from build123d import *

# Parameters (mm, degrees)
SKETCH1_W           = 90
SKETCH1_H           = 30
BOSS_EXTRUDE1_DEPTH = 5.9
SKETCH2_R           = 2.75
CUT_EXTRUDE1_DEPTH  = 10
SKETCH3_W           = 5.9
SKETCH3_H           = 10
CUT_EXTRUDE2_DEPTH  = 10
CUT_EXTRUDE5_REACH  = 7.9
SKETCH6_R           = 2.05
FILLET1_R           = 12
FILLET1_2_R         = 6


with BuildPart() as part:
    # Sketch1 → Boss-Extrude1 (new body)
    with BuildSketch(Plane(origin=(0, 0, 0), x_dir=(1, 0, 0), z_dir=(0, 1, 0))):
        Rectangle(SKETCH1_W, SKETCH1_H)
    extrude(amount=BOSS_EXTRUDE1_DEPTH)

    # Sketch2 → Cut-Extrude1 (cut)
    with BuildSketch(Plane(origin=(0, 5.9, 0), x_dir=(1, 0, 0), z_dir=(0, 1, 0))):
        with Locations((25, 0)):
            Circle(SKETCH2_R)
        with Locations((-38, 0)):
            Circle(SKETCH2_R)
    extrude(amount=-CUT_EXTRUDE1_DEPTH, mode=Mode.SUBTRACT)

    # Sketch3 → Cut-Extrude2 (cut)
    with BuildSketch(Plane(origin=(0, 5.9, 0), x_dir=(1, 0, 0), z_dir=(0, 1, 0))):
        with Locations((-2.95, 0)):
            Rectangle(SKETCH3_W, SKETCH3_H)
    extrude(amount=-CUT_EXTRUDE2_DEPTH, mode=Mode.SUBTRACT)

    # Sketch6 → Cut-Extrude5 (cut, up to next)
    with BuildSketch(Plane(origin=(0, 5.9, 0), x_dir=(1, 0, 0), z_dir=(0, 1, 0)), mode=Mode.PRIVATE) as cut_extrude5_sk1:
        with Locations((0, 5)):
            Circle(SKETCH6_R)
    cut_extrude5_tool1 = extrude(cut_extrude5_sk1.sketch, amount=-CUT_EXTRUDE5_REACH, mode=Mode.PRIVATE) & part.part
    add(cut_extrude5_tool1.solids().sort_by_distance((0, 5.9, -5))[0], mode=Mode.SUBTRACT)
    # Sketch6 → Cut-Extrude5 (cut, up to next)
    with BuildSketch(Plane(origin=(0, 5.9, 0), x_dir=(1, 0, 0), z_dir=(0, 1, 0)), mode=Mode.PRIVATE) as cut_extrude5_sk2:
        with Locations((-5.9, 5)):
            Circle(SKETCH6_R)
    cut_extrude5_tool2 = extrude(cut_extrude5_sk2.sketch, amount=-CUT_EXTRUDE5_REACH, mode=Mode.PRIVATE) & part.part
    add(cut_extrude5_tool2.solids().sort_by_distance((-5.9, 5.9, -5))[0], mode=Mode.SUBTRACT)
    # Sketch6 → Cut-Extrude5 (cut, up to next)
    with BuildSketch(Plane(origin=(0, 5.9, 0), x_dir=(1, 0, 0), z_dir=(0, 1, 0)), mode=Mode.PRIVATE) as cut_extrude5_sk3:
        with Locations((0, -5)):
            Circle(SKETCH6_R)
    cut_extrude5_tool3 = extrude(cut_extrude5_sk3.sketch, amount=-CUT_EXTRUDE5_REACH, mode=Mode.PRIVATE) & part.part
    add(cut_extrude5_tool3.solids().sort_by_distance((0, 5.9, 5))[0], mode=Mode.SUBTRACT)
    # Sketch6 → Cut-Extrude5 (cut, up to next)
    with BuildSketch(Plane(origin=(0, 5.9, 0), x_dir=(1, 0, 0), z_dir=(0, 1, 0)), mode=Mode.PRIVATE) as cut_extrude5_sk4:
        with Locations((-5.9, -5)):
            Circle(SKETCH6_R)
    cut_extrude5_tool4 = extrude(cut_extrude5_sk4.sketch, amount=-CUT_EXTRUDE5_REACH, mode=Mode.PRIVATE) & part.part
    add(cut_extrude5_tool4.solids().sort_by_distance((-5.9, 5.9, 5))[0], mode=Mode.SUBTRACT)

    # Fillet1
    fillet1_edges = [part.edges().sort_by_distance(p)[0] for p in [
        (-45, 2.95, -15),
        (-45, 2.95, 15),
    ]]
    fillet(fillet1_edges, radius=FILLET1_R)

    # Fillet1 2
    fillet1_2_edges = [part.edges().sort_by_distance(p)[0] for p in [
        (45, 2.95, 15),
        (45, 2.95, -15),
    ]]
    fillet(fillet1_2_edges, radius=FILLET1_2_R)


solid = part.part
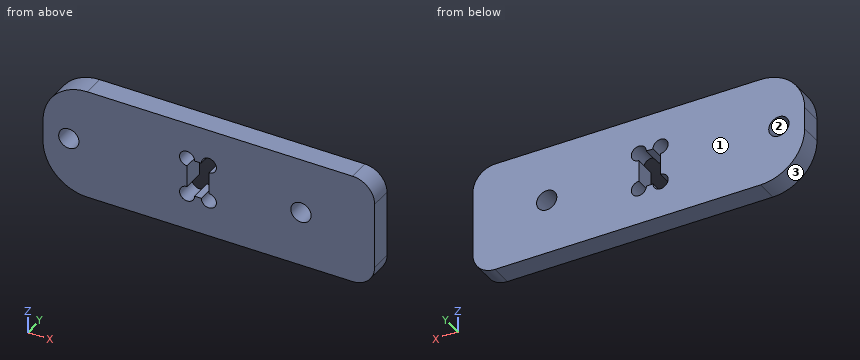
The listing builds one solid part. Answer for the finished solid, in the listing's coordinates (mm). Face numbers are marked on the shaded views. Coordinates: 2 decimals unless noted, no trailing zeros. Write each loop counter-clockwise with the first axis right and the second up, starting at its lowest first coordinate (ties: lowest second). Pieces come first, ordered by that corner, then holes. Notation, with made-up numbers: (-16, 66.5) -> (15, 66.5) arc R17 ccw to (15, 87.5) -> close; hole circle Ø2 at (27.25, -29). An arc over 180 degrees is marked (long way). One line per question, with ' | ' between items.
1. Section B-B (z = 1.5) is taken. Determine the outline of the cut face in (x, y).
Verdict:
outline: (-45, 0) -> (-40.3, 0) -> (-40.3, 5.9) -> (-45, 5.9) -> close; (-35.7, 0) -> (-5.9, 0) -> (-5.9, 5.9) -> (-35.7, 5.9) -> close; (0, 0) -> (22.7, 0) -> (22.7, 5.9) -> (0, 5.9) -> close; (27.3, 0) -> (45, 0) -> (45, 5.9) -> (27.3, 5.9) -> close
2. Section A-A (y = 1.8) is taken. Determine the outline of the cut face in (x, z).
Verdict:
outline: (-45, -3) arc R12 ccw to (-33, -15) -> (39, -15) arc R6 ccw to (45, -9) -> (45, 9) arc R6 ccw to (39, 15) -> (-33, 15) arc R12 ccw to (-45, 3) -> close; hole circle Ø5.5 at (-38, 0); hole (-5.9, -2.95) arc R2.05 ccw (long way) to (-3.85, -5) -> (-2.05, -5) arc R2.05 ccw (long way) to (0, -2.95) -> (0, 2.95) arc R2.05 ccw (long way) to (-2.05, 5) -> (-3.85, 5) arc R2.05 ccw (long way) to (-5.9, 2.95) -> close; hole circle Ø5.5 at (25, 0)
3. Section C-C (x = -38) is taken. Determine the outline of the cut face in (y, z).
Verdict:
outline: (0, -13.91) -> (5.9, -13.91) -> (5.9, -2.75) -> (0, -2.75) -> close; (0, 2.75) -> (5.9, 2.75) -> (5.9, 13.91) -> (0, 13.91) -> close
4. For a pull along Z with two mould halves and no side action, classify the marked faces 1, 2 and 3 as released by +Z, released by -Z, zero draft, split by the parting line, or undercut.
Verdict:
face 1: zero draft | face 2: undercut | face 3: released by -Z
5. Section D-D (z = 6) is taken. Determine the outline of the cut face in (x, y).
Verdict:
outline: (-44.62, 0) -> (-7.69, 0) -> (-7.69, 5.9) -> (-44.62, 5.9) -> close; (-4.11, 0) -> (-1.79, 0) -> (-1.79, 5.9) -> (-4.11, 5.9) -> close; (1.79, 0) -> (45, 0) -> (45, 5.9) -> (1.79, 5.9) -> close
6. Straight lines are drawn through the part: line 1 (X direction, y = 2.85, z = 0); line 2 (X direction, y = 1.95, z = -6.5); line 3 (X direction, y = 3.9, z = -4.5). For each, find the intervals that lie inside material, in ascending order.
Verdict:
line 1: x = -45 to -40.75, -35.25 to -5.9, 0 to 22.25, 27.75 to 45 | line 2: x = -44.48 to -7.3, -4.5 to -1.4, 1.4 to 45 | line 3: x = -44.91 to -7.89, 1.99 to 45
